```python
from build123d import *

# Parameters (mm, degrees)
F1_DEPTH = 76.2
F3_DEPTH = 63.5


with BuildPart() as f1:
    # F0 (on Front) → F1 (new body, symmetric)
    with BuildSketch(Plane.XZ):
        with BuildLine():
            ThreePointArc((3.1831930964, -14.5487436358), (9.9183851872, -17.338551545), (12.7081930964, -24.0737436358))
            Line((12.7081930964, -24.0737436358), (18.0421930964, -24.0737436358))
            Line((18.0421930964, -24.0737436358), (18.0421930964, -9.5957436358))
            Line((18.0421930964, -9.5957436358), (10.9887288065, -0.0582332264))
            Line((10.9887288065, -0.0582332264), (8.9465308884, -1.5685403684))
            Line((8.9465308884, -1.5685403684), (-6.1565405318, 18.8534388128))
            Line((-6.1565405318, 18.8534388128), (-4.1143426137, 20.3637459548))
            Line((-4.1143426137, 20.3637459548), (-11.1678069036, 29.9012563642))
            Line((-11.1678069036, 29.9012563642), (-20.0578069036, 29.9012563642))
            Line((-20.0578069036, 29.9012563642), (-20.0578069036, 17.5822563642))
            add(Edge.make_bspline(
                [(-20.0578069036, 17.5822563642), (-10.1148920839, 15.5647495743), (-12.2363609879, 0.8391823706), (-4.9954212044, -9.7400596384), (3.1831930964, -9.4687436358)],
                knots=[0, 0, 0, 0, 0.513981523, 1, 1, 1, 1], degree=3))
            Line((3.1831930964, -9.4687436358), (3.1831930964, -14.5487436358))
        make_face()
    extrude(amount=F1_DEPTH, both=True)

    # F2 (on Top) → F3 (intersect, symmetric)
    with BuildSketch(Plane.XY):
        Polygon((18.0421930964, 0), (-20.0578069036, 38.1), (-20.0578069036, -38.1), align=None)
    extrude(amount=F3_DEPTH, both=True, mode=Mode.INTERSECT)


solid = f1.part
```
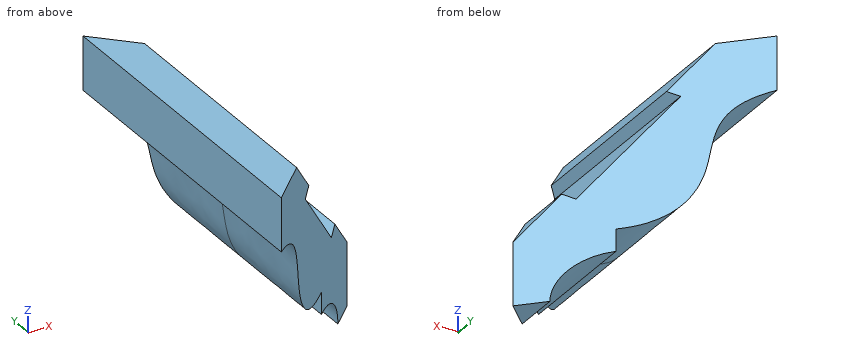
Model file for the job. Use its own axes, mm. Coordinates: 2 decimals unless noted, no trailing zeros. Loops run counter-clockwise (first coordinate to the right, second up) from the corner with the lowest first, then second, coordinate; pieces in that order, holes last. Notation, with made-up numbers: (63.25, -37.75) - (79.25, -37.75) arc R22 ccw to (79.25, -8.75) - close; hole circle Ø10 at (45, 20.5). An arc over 180 degrees is marked (long way). Write item = value, one per line. Start each with the question number.
Item 1: Wall check: probe 1 along Z at (x, y) = (-5.5, -15); probe 2 along Y at (x, z) = (-7, 13); probe 3 along Y at (x, z) = (-11.5, 14). Give the ranges that are in metal, low to high. Write a range as [from, to].
Item 2: Saw through at A-A, the plane z = -13.5. List the corners of the cut face in (x, y).
Item 3: Saw through at B-B, the plane x = 5.5. List the corners of the cut face in (y, z).
Item 4: Drop flat-ended pins along their axis: pin 1 Ø1 at (x, z) = (14, -9.5) entering from -Y; pin 2 Ø12 at (y, z) = (-25.5, -17) entering from +X; pin 3 Ø4 at (x, y) = (-0.5, 13) entering from +Z; pin 4 Ø4 at (y, z) = (1, 12.5) entering from -X. Give the stop position or say it passes through.
Item 5: Saw through at C-C, the plane z = 24. List the corners of the cut face in (x, y), then the cut area to 3 significant figures.
Answers:
q1.probe_1 = [-6.74, 17.97], [19.34, 22.24]
q1.probe_2 = [-25.04, 25.04]
q1.probe_3 = [-29.54, 29.54]
q2.outline = (3.18, -14.86) - (18.04, 0) - (3.18, 14.86) - close
q3.outline = (-12.54, -14.83) - (12.54, -14.83) - (12.54, 3.09) - (-12.54, 3.09) - close
q4.pin_1 = -4.54
q4.pin_2 = through
q4.pin_3 = 13.91
q4.pin_4 = -13.77
q5.outline = (-20.06, -38.1) - (-6.8, -24.85) - (-6.8, 24.85) - (-20.06, 38.1) - close
q5.area = 834 mm2
